```python
from build123d import *

# Parameters (mm, degrees)
ESBO_O1_R                = 3.5
RESSALTO_EXTRUS_O1_DEPTH = 10
ESBO_O2_R                = 3.5
CORTE_EXTRUS_O1_DEPTH    = 10
ESBO_O3_W                = 13
ESBO_O3_H                = 18.5
CORTE_EXTRUS_O2_DEPTH    = 10


with BuildPart() as part:
    # Esboço1 → Ressalto-extrusão1 (new, symmetric)
    with BuildSketch(Plane(origin=(0, 0, 0), x_dir=(0, 0, -1), z_dir=(1, 0, 0))):
        with BuildLine():
            Line((-6.5, 0), (-6.5, -22))
            Line((-6.5, -22), (6.5, -22))
            Line((6.5, -22), (6.5, 0))
            ThreePointArc((6.5, 0), (0, 6.5), (-6.5, 0))
        make_face()
        Circle(ESBO_O1_R, mode=Mode.SUBTRACT)
    extrude(amount=RESSALTO_EXTRUS_O1_DEPTH, both=True)

    # Esboço2 → Corte-extrusão1 (cut, symmetric)
    with BuildSketch(Plane.XY):
        with Locations(Location((0, -17, 0), (0, 0, 270))):
            Circle(ESBO_O2_R)
    extrude(amount=CORTE_EXTRUS_O1_DEPTH, both=True, mode=Mode.SUBTRACT)

    # Esboço3 → Corte-extrusão2 (cut, symmetric)
    with BuildSketch(Plane.XY):
        with Locations((0, -2.75)):
            Rectangle(ESBO_O3_W, ESBO_O3_H)
    extrude(amount=CORTE_EXTRUS_O2_DEPTH, both=True, mode=Mode.SUBTRACT)


solid = part.part
```
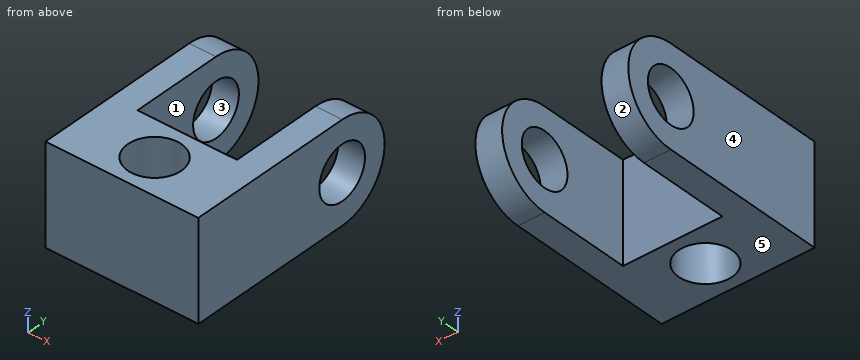
Part model, mm, in its own coordinate system. Face numbers are marked on the shaded views. A direction names the side the tool comes from. Round coordinates to 2 decimals unless told otherwise and drop trailing zeros. Order: outer loops, then holes, each group sorted by start corner. A loop starts at its lowest first (then second) coordinate and runs counter-clockwise, first axis right, second up. Notation, with made-up numbers: M 17.5,10.5 L 59.5,10.5 A32 ccw 59.5,44.5 Z; hole C -5.75,84.5 d7. An arc over 180 degrees is marked long. Answer in a Markdown table with one row per item. Add a question column.
Q1. Cut at D-D on y = 0.5. Give the cut face in (x, z).
Q2. Cut at C-C on y = -10.25. Give the cut face in (x, z), and give its area (3 significant figures).
Q3. Cut at A-A on z = 0. Give the cut face in (x, y), and give its area (3 significant figures).
Q4. Pin check, flat tip, straight feed: pin 1 (3 mm diameter, centred on x = -1, z = 3.5, fed in from +Y). Stop position of the tip, or through.
Q5. Wall check: L1, parallel to Y at x = -9.3, z = 0; L2, parallel to X at y = 3.5, z = -1.25; L3, parallel to X at y = -17, z = -2.75. Give the ranges that are in metal, low to high. Write a range as from..to.
Q6. 3-axis set-ups, long thin cutter, end or side, ignore diameter. For the marked faces 1 and 2: which of +Z, -Z, +X, -X, +Y, -Y reach the whole face in a straight line?
Q7. Mould opens along Z. For the marked faces 3, 4 and 5 say: +Z half, -Z half, draft (parallel to the pull), parting line (faces both ways), or undercut.
Q8. Cut at B-B on x = 0. Give the cut face in (y, z), and give its area (3 significant figures).
Established:
| question | item | result |
|---|---|---|
| 1 | outline | M -10,-6.48 L -6.5,-6.48 L -6.5,-3.46 L -10,-3.46 Z; M -10,3.46 L -6.5,3.46 L -6.5,6.48 L -10,6.48 Z; M 6.5,-6.48 L 10,-6.48 L 10,-3.46 L 6.5,-3.46 Z; M 6.5,3.46 L 10,3.46 L 10,6.48 L 6.5,6.48 Z |
| 2 | outline | M -10,-6.5 L -6.5,-6.5 L -6.5,6.5 L -10,6.5 Z; M 6.5,-6.5 L 10,-6.5 L 10,6.5 L 6.5,6.5 Z |
| 2 | area | 91.0 mm2 |
| 3 | outline | M -10,-22 L 10,-22 L 10,-3.5 L 6.5,-3.5 L 6.5,-12 L -6.5,-12 L -6.5,-3.5 L -10,-3.5 Z; M -10,3.5 L -6.5,3.5 L -6.5,6.5 L -10,6.5 Z; M 6.5,3.5 L 10,3.5 L 10,6.5 L 6.5,6.5 Z; hole C 0,-17 d7 |
| 3 | area | 242 mm2 |
| 4 | pin 1 | stops at y = -12 |
| 5 | L1 | y = -22..-3.5, 3.5..6.5 |
| 5 | L2 | x = -10..-6.5, 6.5..10 |
| 5 | L3 | x = -10..-3.5, 3.5..10 |
| 6 | face 1 | +Z, -Z, +Y |
| 6 | face 2 | +X, -X, +Y |
| 7 | face 3 | undercut |
| 7 | face 4 | draft |
| 7 | face 5 | -Z half |
| 8 | outline | M -22,-6.5 L -20.5,-6.5 L -20.5,6.5 L -22,6.5 Z; M -13.5,-6.5 L -12,-6.5 L -12,6.5 L -13.5,6.5 Z |
| 8 | area | 39.0 mm2 |
